Could you check a few things on this model? Use its own coordinates, in mm. A direction names the side the tool comes from. Round coordinates to 2 decimals unless told otherwise and drop trailing zeros. Loops run counter-clockwise (first coordinate to the right, second up) from the corner with the lowest first, then second, coordinate; pieces in that order, holes last. Notation, with made-up numbers: (13.5, 38.5) -> (71.5, 38.5) arc R19 ccw to (71.5, 43.5) -> close; hole circle Ø3 at (-3.75, 37). An arc over 180 degrees is marked (long way). One line per item, written item: value.
Autodesk Inventor part; units mm, degrees
ref_plane "YZ Plane" through (0, 0, 0) normal (1, 0, 0) x (0, 1, 0)
ref_plane "XZ Plane" through (0, 0, 0) normal (0, 1, 0) x (-1, 0, 0)
ref_plane "XY Plane" through (0, 0, 0) normal (0, 0, 1) x (1, 0, 0)
sketch "Sketch1" plane through (0, 0, 0) normal (0, 1, 0) x (-1, 0, 0)
  line L0 (39.6667, 0.3125) -> (0, 37.5)
  line L1 (0, 37.5) -> (5, 37.5)
  line L2 (5, 37.5) -> (39.6667, 5)
  line L3 (39.6667, 5) -> (39.6667, 0.3125)
  point P0 (0, 0)
  dimension "d2" = 5
  dimension "d46" = 32.5
extrude "Extrusion1" add sketch "Sketch1" along normal blind 70
sketch "Sketch2" plane through (-39.6667, 0, 0.3125) normal (0.6839, 0, -0.7295) x (-0.7295, 0, -0.6839)
  line L0 (-54.3406, 0) -> (-29.3406, 0)
  line L1 (-29.3406, 0) -> (-34.3406, 0)
  line L2 (-34.3406, 0) -> (-24.3406, 0)
  line L3 (-28.7246, 0) -> (-30.2246, 0)
  line L4 (-30.2246, 0) -> (-30.2246, 8)
  line L5 (-30.2246, 8) -> (-32.2246, 8)
  line L6 (-32.2246, 8) -> (-32.2246, 13)
  line L7 (-32.2246, 13) -> (-25.2246, 13)
  line L8 (-25.2246, 13) -> (-25.2246, 8)
  line L9 (-25.2246, 8) -> (-27.2246, 8)
  line L10 (-27.2246, 8) -> (-27.2246, 0)
  line L11 (-54.3406, 0) -> (-54.3406, 35)
  line L12 (-54.3406, 35) -> (0.1481, 35)
  line L13 (0.1481, 35) -> (0.1481, 0)
  line L14 (-29.3406, 70) -> (-34.3406, 70)
  line L15 (-34.3406, 70) -> (-24.3406, 70)
  line L16 (-28.7246, 70) -> (-30.2246, 70)
  line L17 (-30.2246, 70) -> (-30.2246, 62)
  line L18 (-30.2246, 62) -> (-32.2246, 62)
  line L19 (-32.2246, 62) -> (-32.2246, 57)
  line L20 (-32.2246, 57) -> (-25.2246, 57)
  line L21 (-25.2246, 57) -> (-25.2246, 62)
  line L22 (-25.2246, 62) -> (-27.2246, 62)
  line L23 (-27.2246, 62) -> (-27.2246, 70)
  dimension "d7" = 25
  dimension "d8" = 5
  dimension "d9" = 10
  dimension "d10" = 1.5
  dimension "d11" = 8
  dimension "d12" = 2
  dimension "d13" = 5
  dimension "d14" = 7
  dimension "d15" = 2
  dimension "d16" = 35
extrude "Extrusion2" cut sketch "Sketch2" against normal blind 5 contours L4 L5 L6 L7 L8 L9 L10 L2 L0
extrude "Extrusion3" cut sketch "Sketch2" against normal blind 5 contours L15 L23 L22 L21 L20 L19 L18 L17 L14
sketch "Sketch3" plane through (0, 70, 0) normal (0, 1, 0) x (1, 0, 0)
  line L0 (0, -37.4883) -> (-7.9979, -29.936)
  line L1 (0, -37.4883) -> (-5.022, -37.4883)
  line L2 (-5.022, -37.4883) -> (-45.0001, 0)
  line L3 (0, -37.4883) -> (-7.9979, -29.936)
  line L4 (-7.9979, -29.936) -> (-10.3827, -32.4615)
  line L5 (-10.3827, -32.4615) -> (-16.9476, -26.3054)
  line L6 (-21.8663, -16.9314) -> (-24.2422, -19.4651)
  line L7 (-24.2422, -19.4651) -> (-31.5368, -12.6248)
  line L8 (-31.5368, -12.6248) -> (-29.1608, -10.0911)
  line L9 (-21.8663, -16.9314) -> (-29.1608, -10.0911)
  line L10 (-10.3827, -32.4615) -> (-17.6772, -25.6212)
  line L11 (-7.9979, -29.936) -> (-21.8663, -16.9314)
  line L12 (-17.6772, -25.6212) -> (-15.3013, -23.0875)
  point P0 (0, 0)
  dimension "d25" = 90
  dimension "d28" = 10
  dimension "d32" = 18.4566
  dimension "d33" = 10
extrude "Extrusion4" add sketch "Sketch3" along normal blind 5 contours L4 L2 L12 L11 | L6 L2 L8 L9
sketch "Sketch4" plane through (0, 0, 0) normal (0, -1, 0) x (1, 0, 0)
  line L0 (0.1144, 37.3726) -> (-7.596, 30.2452)
  line L1 (0.1144, 37.3726) -> (-4.8856, 37.3726)
  line L2 (-4.8856, 37.3726) -> (-44.8855, -0.1225)
  line L3 (-4.8856, 37.3726) -> (-9.8845, 32.6867)
  line L4 (-7.596, 30.2452) -> (-9.8845, 32.6867)
  line L5 (-9.8845, 32.6867) -> (-17.1803, 25.8478)
  line L6 (-17.1803, 25.8478) -> (-14.9244, 23.4411)
  line L7 (-14.9244, 23.4411) -> (-22.2202, 16.6022)
  line L8 (-22.2202, 16.6022) -> (-24.4761, 19.0088)
  line L9 (-24.4761, 19.0088) -> (-31.7719, 12.1699)
  line L10 (-31.7719, 12.1699) -> (-29.6284, 9.8832)
  line L11 (-29.6284, 9.8832) -> (-29.549, 9.7985)
  line L12 (-29.549, 9.7985) -> (-29.5486, 9.7981)
  line L13 (-29.5486, 9.7981) -> (-22.2202, 16.6022)
  line L14 (-14.9244, 23.4411) -> (-7.596, 30.2452)
  point P0 (0, 0)
extrude "Extrusion5" add sketch "Sketch4" along normal blind 5 contours L14 L6 L2 L4 | L13 L11 L10 L2 L8
properties part number "lat_front_mdf2"
Item 1: Will these pins go through, and if not, where does the flat tip stop? pin 1 Ø3 at (x, z) = (-35, 6) entering from +Y; pin 2 Ø4 at (y, z) = (63.5, 30.5) entering from -X; pin 3 Ø8 at (x, z) = (-19.5, 15) entering from -Y; pin 4 Ø3 at (x, z) = (-18, 22) entering from -Y.
Output:
pin 1: stops at y = 70
pin 2: stops at x = -14.6
pin 3: stops at y = -5
pin 4: stops at y = 0
Item 2: I need wall thicknesses on line 1 (Y direction, x = -22.5, z = 18.5); line 2 (Z direction, x = -2, y = 62.5) (3 decimals); line 3 (X direction, y = 57, z = 33). Which ranges of each line are inside material? Lowest first, please. Write a range as from..to.
Output:
line 1: y = 0..70
line 2: z = 35.625..37.5
line 3: x = -9.8..-4.8
Item 3: If we section it at D-D on x = -9: List the corners of the cut face in (y, z) for me, plus the area to 3 significant figures.
Output:
outline: (-5, 28.94) -> (0, 28.94) -> (0, 29.06) -> (70, 29.06) -> (70, 29) -> (75, 29) -> (75, 31) -> (70, 31) -> (70, 33.75) -> (0, 33.75) -> (0, 31.74) -> (-5, 31.74) -> close
area: 352 mm²
Item 4: If we section it at A-A on y = 60: List the corners of the cut face in (x, z) for me, plus the area to 3 significant figures.
Output:
outline: (-39.67, 0.31) -> (-21.26, 17.56) -> (-23.6, 20.06) -> (-39.67, 5) -> close; (-18.5, 24.85) -> (-16.16, 22.35) -> (0, 37.5) -> (-5, 37.5) -> close
area: 150 mm²
Item 5: If we mould it in two halves opening along Y, with no side actions, what happens to faces 1 (the face through (-2, 35, 37.5)), 2 (the face through (-18, 8, 23)), 3 (the face through (-22, 70, 19))? For each: released by +Y, released by -Y, zero draft, split by the parting line, or undercut.
Output:
face 1: zero draft
face 2: undercut
face 3: released by +Y
Item 6: For faces 4 (the face through (-27.84, 72.46, 16.09)), 5 (the face through (-13, 75, 28)), 6 (the face through (-35, 70, 6)), 7 (the face through (-18, 62, 23)), which set-ups out of +Z, -Z, +X, -X, +Y, -Y let a thin tool reach every point of the face, with its end or its side?
Output:
face 4: +Z, -X, +Y, -Y
face 5: +Z, -Z, +X, -X, +Y
face 6: -Z, -X, +Y
face 7: -Z, -X
Item 7: If we section it at C-C on y = 38: List the corners of the cut face in (x, z) for me.
Output:
outline: (-39.67, 0.31) -> (0, 37.5) -> (-5, 37.5) -> (-39.67, 5) -> close
